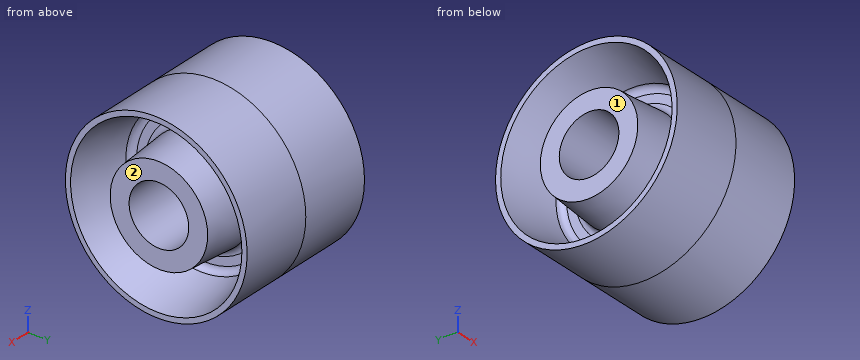
```python
from build123d import *

# Parameters (mm, degrees)
FILLET4_R = 3
FILLET5_R = 3


with BuildPart() as part:
    # Sketch1 → Revolve1 (revolve)
    with BuildSketch(Plane.XY):
        Polygon((0, 13.45), (0, 41), (33, 41), (33, 38.639986999), (6, 33), (6, 24), (31.5, 22), (31.5, 13.45), align=None)
    revolve(axis=Axis((-113.627257408, 0, 0), (1, 0, 0)))

    # Fillet4
    fillet4_edges = [part.edges().sort_by_distance(p)[0] for p in [
        (6, -33, 0),
    ]]
    fillet(fillet4_edges, radius=FILLET4_R)

    # Fillet5
    fillet5_edges = [part.edges().sort_by_distance(p)[0] for p in [
        (6, -24, 0),
    ]]
    fillet(fillet5_edges, radius=FILLET5_R)

    # Mirror1: part across plane


with BuildPart() as part_1:
    add(part.part)
    add(part.part.mirror(Plane(origin=(0, 0, 0), x_dir=(0, 0, 1), z_dir=(1, 0, 0))))


solid = part_1.part
```
Can you work these out from the model? Positions are in its coordinate system, mm. Face numbers are marked on the shaded views. A direction names the side the tool comes from. Coordinates: 2 decimals unless noted, no trailing zeros. Order: outer loops, then holes, each group sorted by start corner. A loop starts at its lowest first (then second) coordinate and runs counter-clockwise, first axis right, second up.
1. I need wall thicknesses on line 1 (Z direction, x = 29, y = 5); line 2 (Y direction, x = 18, z = -14.5); line 3 (Y direction, x = -22, z = 2). Which ranges of each line are inside material? Lowest first, please.
2. If we section it at C-C (x = 4): Please give me the cut outline in (y, z).
3. I'm going to push flat-ended pins straight in: pin 1 (4 mm diameter, centred on x = 12, z = -17, fed in from -Y); pin 2 (6 mm diameter, centred on y = -21, z = -5.5, fed in from +X); pin 3 (3 mm diameter, centred on x = -22.5, y = 24, fed in from +Z); pin 4 (16 mm diameter, centred on y = 0, z = 0, fed in from +X). Where does each tip first touch, or does it pass through?
4. For the marked faces 1 and 2, which set-ups out of +Z, -Z, +X, -X, +Y, -Y let a thin tool reach every point of the face, with its end or its side?
5. If we section it at D-D (x = 18.5): Please give me the cut outline in (y, z).
Entries:
1. line 1: z = -40.69 to -37.47, -21.63 to -12.49, 12.49 to 21.63, 37.47 to 40.69
1. line 2: y = -38.35 to -32.41, -17.93 to 17.93, 32.41 to 38.35
1. line 3: y = -40.95 to -36.29, -22.66 to -13.3, 13.3 to 22.66, 36.29 to 40.95
2. outline: circle Ø82 at (0, 0); hole circle Ø26.9 at (0, 0)
3. pin 1: stops at y = -38.16
3. pin 2: stops at x = 31.5
3. pin 3: stops at z = 34.27
3. pin 4: passes through
4. face 1: -X
4. face 2: +X
5. outline: circle Ø82 at (0, 0); circle Ø46.04 at (0, 0); hole circle Ø71.22 at (0, 0); hole circle Ø26.9 at (0, 0)
